from build123d import *

# Parameters (mm, degrees)
CROQUIS1_W              = 101.6
CROQUIS1_H              = 68.58
SALIENTE_EXTRUIR1_DEPTH = 17.78
CROQUIS4_W              = 41.061151145
CROQUIS4_H              = 91.44
SALIENTE_EXTRUIR2_DEPTH = 14.224
CORTAR_EXTRUIR1_DEPTH   = 6.35
REDONDEO2_R             = 3.048
CORTAR_EXTRUIR2_DEPTH   = 160.707882909


with BuildPart() as part:
    # Croquis1 → Saliente-Extruir1 (new body)
    with BuildSketch(Plane(origin=(0, 0, 0), x_dir=(1, 0, 0), z_dir=(0, 1, 0))):
        with Locations((50.8, 34.29)):
            Rectangle(CROQUIS1_W, CROQUIS1_H)
    extrude(amount=SALIENTE_EXTRUIR1_DEPTH)

    # Croquis4 → Saliente-Extruir2 (add)
    with BuildSketch(Plane(origin=(3.692565329, -7.385130657, -6.395710759), x_dir=(-0.8660254037844416, 0, -0.49999999999999484), z_dir=(-0.3535533905932708, 0.7071067811865462, 0.6123724356957978))):
        with Locations((-23.148130824, -81.308869074)):
            Rectangle(CROQUIS4_W, CROQUIS4_H)
    extrude(amount=-SALIENTE_EXTRUIR2_DEPTH)

    # Croquis5 → Cortar-Extruir1 (cut)
    with BuildSketch(Plane(origin=(3.692565329, -7.385130657, -6.395710759), x_dir=(0.9354143466934866, 0.2672612419124214, 0.23145502494313694), z_dir=(-0.35355339059327084, 0.707106781186546, 0.612372435695798))):
        with BuildLine():
            Line((60.564352246, 112.481567013), (78.322456444, 105.231851332))
            Line((78.322456444, 105.231851332), (52.267557185, 41.410642848))
            ThreePointArc((52.267557185, 41.410642848), (39.763647245, 36.156448589), (34.509452987, 48.660358529))
            Line((34.509452987, 48.660358529), (60.564352246, 112.481567013))
        make_face()
    extrude(amount=-CORTAR_EXTRUIR1_DEPTH, mode=Mode.SUBTRACT)

    # Redondeo2
    redondeo2_edges = [part.edges().sort_by_distance(p)[0] for p in [
        (46.379886856, 17.78, -34.036058837),
    ]]
    fillet(redondeo2_edges, radius=REDONDEO2_R)

    # Croquis6 → Cortar-Extruir2 (cut, through all)
    with BuildSketch(Plane(origin=(101.6, 0, 0), x_dir=(0, 0, -1), z_dir=(1, 0, 0))):
        Polygon((6.096, 9.398), (39.624, 9.398), (34.19806217, 0), (11.52193783, 0), align=None)
    extrude(amount=-CORTAR_EXTRUIR2_DEPTH, mode=Mode.SUBTRACT)


solid = part.part
Design review of the part built by this model. Coordinates are the model's own, in mm. A direction names the side the tool comes from. Give positions to 0.01 mm unless a question says otherwise; leave off trailing zeros. Loops run counter-clockwise (first coordinate to the right, second up) from the corner with the lowest first, then second, coordinate; pieces in that order, holes last. Notation, with made-up numbers: M -1.5,13.25 L 4.5,13.25 A35 ccw 4.5,51.25 Z; hole C -21,88 d9. An arc over 180 degrees is marked long. Write item = value, one per line.
Q1. We need section A-A (x = 14.5). Give the boundary of the cut face in (y, z).
Output values:
outline = M 0,-68.58 L 17.78,-68.58 L 17.78,0 L 0,0 L 0,-11.52 L 9.4,-6.1 L 9.4,-39.62 L 0,-34.2 Z
Q2. Draft analysis for pull direction Y (two halves, no side actions). For faces 6 (the cylindrical face through (42.178, 24.7, -26.337)), 7 (the flat face through (66.048, 56.193, -48.921)), 8 (the flat face through (61.41, 47.34, -59.49)), state which applies: +Y half, -Y half, draft (parallel to the pull), parting line (faces both ways), or undercut.
Output values:
face_6 = +Y half
face_7 = draft
face_8 = undercut
Q3. Insertion check: pin 1 (20.5 mm diameter, centred on x = 26, z = -19.5, fed in from +Y); pin 2 (3 mm diameter, centred on x = 55, y = 41.5, fed in from -Z); pin 3 (10 mm diameter, centred on x = 67, z = -26, fed in from -Y). Each pin has a flat end and moves straight along its axis. Give the tip position at first contact, or say it passes through.
Output values:
pin_1 = 25.37
pin_2 = -58.39
pin_3 = 9.4
Q4. We need section C-C (z = -66). Give the boundary of the cut face in (x, y), plus the area to 3 significant figures.
Output values:
outline = M 0,0 L 101.6,0 L 101.6,17.78 L 0,17.78 Z; M 41.13,42.84 L 88.54,66.54 L 88.54,78.22 L 80.1,82.44 L 75.91,80.34 L 75.91,71.36 L 53.76,60.29 L 53.76,69.27 L 41.13,62.95 Z
area = 2,530 mm^2
Q5. We need section B-B (y = 5). Give the boundary of the cut face in (x, z).
Output values:
outline = M 0,-68.58 L 101.6,-68.58 L 101.6,-37.08 L 0,-37.08 Z; M 0,-8.64 L 101.6,-8.64 L 101.6,0 L 0,0 Z
Q6. For faces 1 (the flat face through (49.095, 55.511, -57.921)), 2 (the flat face through (37.556, 45.315, -59.813)), 3 (the flat face through (58.669, 51.964, -53.555)), 4 (the flat face through (50, 9, -68.58)), 5 (the flat face through (52, 9.398, -23)), list the 3-axis set-ups (+Z, -Z, +X, -X, +Y, -Y) from which the entire face can be reached by the end or side of a thin tool; tool diameter is ignored.
Output values:
face_1 = +Z, +Y
face_2 = -Z, -X, +Y
face_3 = +Y
face_4 = -Z, +X, -X, -Y
face_5 = +X, -X
Q7. We need section D-D (y = 74.5). Give the boundary of the cut face in (x, z).
Output values:
outline = M 46.9,-76 L 54.84,-89.75 L 90.4,-69.22 L 82.46,-55.47 L 72.99,-60.94 L 77.48,-68.72 L 60.87,-78.31 L 56.38,-70.53 Z
Q8. To check wall thickness, follow line 1 (Y direction, x = 75.5, z = -13); line 2 (Y direction, x = 76.5, z = -6); line 3 (Y direction, x = 82.5, z = -10.5). State the ranges of each line that lie inside material, in increasing order. Write a range as [from, to].
Output values:
line_1 = [9.4, 17.78]
line_2 = [0, 17.78]
line_3 = [0, 1.77], [9.4, 17.78]
